The figure shows three views and two pictorial views of one solid part (mm, origin at its lowest corner). Answer the questions. A direction names the side the tool comes from. Coordinates: 2 decimals unless noted, no trailing zeros. Write each loop counter-clockwise with the first axis right and the second up, starting at its lowest first coordinate (ties: lowest second). Pieces come first, ordered by that corner, then holes. Notation, with made-up numbers: M 8.5,20.5 L 40.5,20.5 A10 ccw 40.5,32.5 Z; hole C -8,65 d1. An arc over 180 degrees is marked long. Answer as CSV lines item,"result".
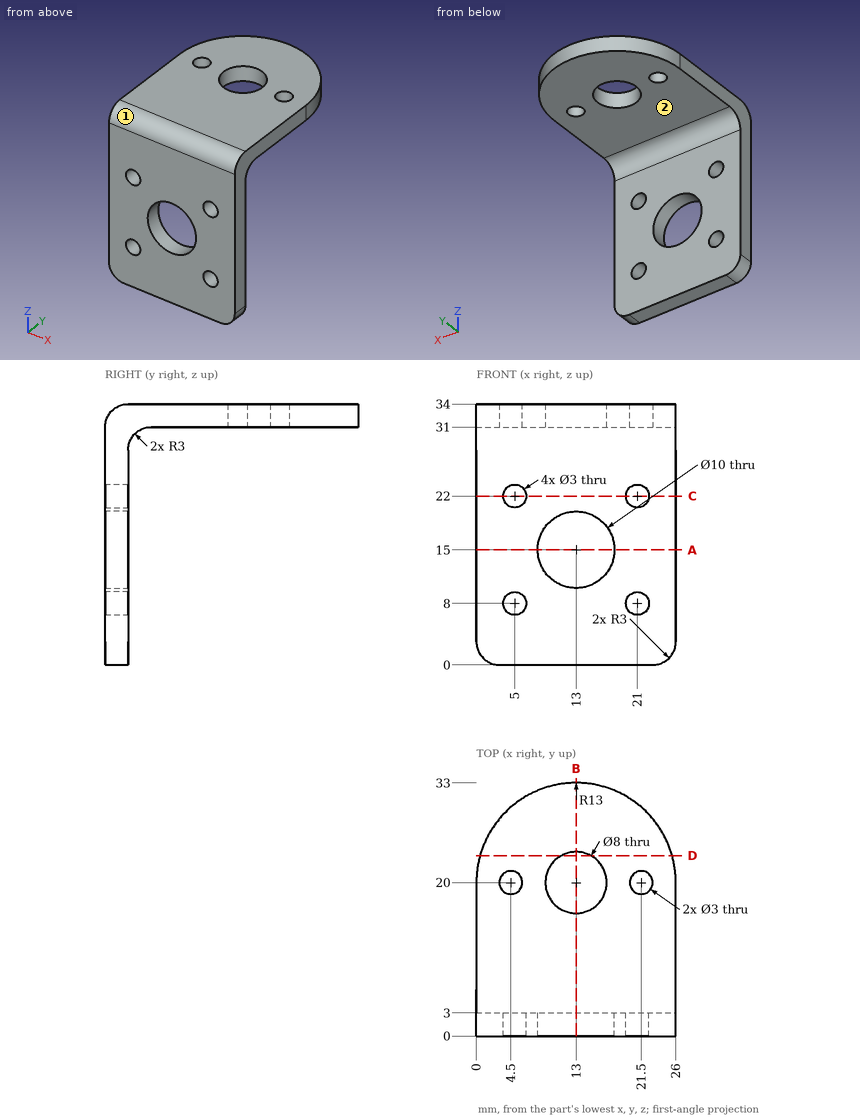
Q1. Straight lines are drawn through the part: line 1 (Z direction, x = 7, y = 27); line 2 (Y direction, x = 21.5, z = 20.5); line 3 (Y direction, x = 13, z = 32.3). For each, find the intervals that lie inside material, in ascending order.
Output:
line 1,"31 to 34"
line 2,"0 to 3"
line 3,"0.3 to 16, 24 to 33"
Q2. Find section D-D (y = 23.5). Give the vertices of the cut face in (x, z), and give its area (3 significant figures).
Output:
outline,"M 0.48,31 L 11.06,31 L 11.06,34 L 0.48,34 Z; M 14.94,31 L 25.52,31 L 25.52,34 L 14.94,34 Z"
area,"63.5 mm2"
Q3. Find section C-C (z = 22). Give the vertices of the cut face in (x, y).
Output:
outline,"M 0,0 L 3.5,0 L 3.5,3 L 0,3 Z; M 6.5,0 L 19.5,0 L 19.5,3 L 6.5,3 Z; M 22.5,0 L 26,0 L 26,3 L 22.5,3 Z"
Q4. Find section B-B (x = 13). Give the vertices of the cut face in (y, z), and give its area (3 significant figures).
Output:
outline,"M 0,0 L 3,0 L 3,10 L 0,10 Z; M 0,20 L 3,20 L 3,28 A3 cw 6,31 L 16,31 L 16,34 L 3,34 A3 ccw 0,31 Z; M 24,31 L 33,31 L 33,34 L 24,34 Z"
area,"138 mm2"
Q5. Find section A-A (z = 15). Give the vertices of the cut face in (x, y).
Output:
outline,"M 0,0 L 8,0 L 8,3 L 0,3 Z; M 18,0 L 26,0 L 26,3 L 18,3 Z"
Q6. For the marked faces 1 and 2, determine the directions among +Z, -Z, +X, -X, +Y, -Y from which every point of the face is accessible in a straight line to the end or side of a thin tool.
Output:
face 1,"+Z, +X, -X, -Y"
face 2,"-Z, +X, -X, +Y"
Q7. Flat-ended cylindrical pins translate along their axes: pin 1 Ø2.5 at (x, z) = (5, 22) entering from -Y; pin 2 Ø1.5 at (x, y) = (7, 14.5) entering from -Z; pin 3 Ø13 at (x, z) = (14.5, 14.5) entering from +Y. Find the tip coordinate at first contact, or state that the pin passes through.
Output:
pin 1,"through"
pin 2,"z = 31"
pin 3,"y = 3"
